from build123d import *

# Parameters (mm, degrees)
F0_R     = 2.15265
F0_R_2   = 3.175
F0_R_3   = 3.660757
F0_R_4   = 1.7272
F0_R_5   = 6.35
F1_DEPTH = 5.08


with BuildPart() as f1:
    # F0 (on Top) → F1 (new body)
    with BuildSketch(Plane.XY):
        with BuildLine():
            Line((0, 22.225), (-264.908055, 22.225))
            Line((-264.908055, 22.225), (-264.908055, -117.625774))
            Line((-264.908055, -117.625774), (22.225, -117.625774))
            Line((22.225, -117.625774), (22.225, -96.670774))
            Line((22.225, -96.670774), (22.225, 0))
            ThreePointArc((22.225, 0), (15.715448, 15.715448), (0, 22.225))
        make_face()
        with Locations((-247.445555, -107.148274)):
            Circle(F0_R, mode=Mode.SUBTRACT)
        with Locations((-260.145555, -90.638274)):
            Circle(F0_R, mode=Mode.SUBTRACT)
        with Locations((7.9375, -107.148274)):
            Circle(F0_R, mode=Mode.SUBTRACT)
        with Locations((-260.145555, 17.4625)):
            Circle(F0_R, mode=Mode.SUBTRACT)
        with Locations((17.4625, -34.548124)):
            Circle(F0_R_2, mode=Mode.SUBTRACT)
        with Locations((-21.328108, -21.328108)):
            Circle(F0_R_2, mode=Mode.SUBTRACT)
        with Locations((-30.356012, -9.164019)):
            Circle(F0_R_3, mode=Mode.SUBTRACT)
        with Locations((-11.786586, -11.786586)):
            Circle(F0_R_4, mode=Mode.SUBTRACT)
        with Locations((11.786586, -11.786586)):
            Circle(F0_R_4, mode=Mode.SUBTRACT)
        Circle(F0_R_5, mode=Mode.SUBTRACT)
        with Locations((-34.548124, 17.4625)):
            Circle(F0_R_2, mode=Mode.SUBTRACT)
        with Locations((-11.786586, 11.786586)):
            Circle(F0_R_4, mode=Mode.SUBTRACT)
        with Locations((11.786586, 11.786586)):
            Circle(F0_R_4, mode=Mode.SUBTRACT)
    extrude(amount=F1_DEPTH)


solid = f1.part
Work out the finished part from the listing and answer in its coordinate system (mm). Round coordinates to 2 decimals unless told otherwise and drop trailing zeros. One line per question, with ' | ' between items. Start each with the question number.
(1) A flat-ended cylindrical pin translates along its axis: pin 1 Ø7.5 at (x, y) = (17.46, -34.55) entering from +Z. Find the tip coordinate at first contact, or state that the pin passes through.
(2) For a pull along X with two mould halves and no side action, classify faces 1 (the face through (-123, -117.626, 3)), 2 (the face through (-18.395, -22.544, 2.504)), 3 (the face through (22.225, -60, 3)) as released by +X, released by -X, zero draft, split by the parting line, or undercut.
(3) Find the intervals of material crossed by line 1 (X direction, y = -11, z = 0.25) (3 decimals); line 2 (Y direction, x = -21, z = 2.65) (3 decimals); line 3 (X direction, y = -1, z = 0.6) (3 decimals), in increasing order.
Geometry check:
1) pin 1: stops at z = 5.08
2) face 1: zero draft | face 2: undercut | face 3: released by +X
3) line 1: x = -264.908 to -33.523, -27.189 to -13.324, -10.249 to 10.249, 13.324 to 22.225 | line 2: y = -117.626 to -24.486, -18.17 to 22.225 | line 3: x = -264.908 to -6.271, 6.271 to 22.225
